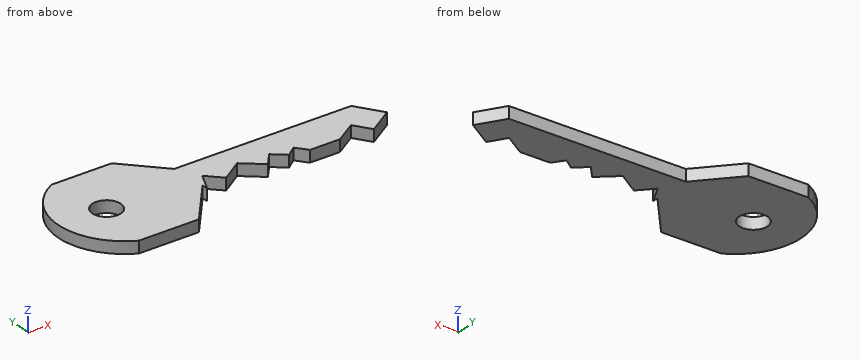
from build123d import *

# Parameters (mm, degrees)
F1_DEPTH = 2.5
F2_R     = 3
F3_DEPTH = 25


with BuildPart() as f1:
    # F0 (on Top) → F1 (new body)
    with BuildSketch(Plane.XY):
        with BuildLine():
            Line((18.500206, 13.484339), (5.681507, 13.484339))
            ThreePointArc((5.681507, 13.484339), (-2.025628, 0.984339), (5.681507, -11.515661))
            Line((5.681507, -11.515661), (18.500206, -11.515661))
            Line((18.500206, -11.515661), (26.226566, -2.179502))
            Line((26.226566, -2.179502), (26.226566, -3.515661))
            Line((26.226566, -3.515661), (28.245927, 0.636009))
            Line((28.245927, 0.636009), (31.124004, -2.351236))
            Line((31.124004, -2.351236), (35.732787, 0.682989))
            Line((35.732787, 0.682989), (39.747892, -2.72324))
            Line((39.747892, -2.72324), (42.058162, 0))
            Line((42.058162, 0), (44.656219, -2.204071))
            Line((44.656219, -2.204071), (46.799748, -0.583421))
            Line((46.799748, -0.583421), (48.568681, -2.923074))
            Line((48.568681, -2.923074), (54.981848, -2.923074))
            Line((54.981848, -2.923074), (59.484062, 0))
            Line((59.484062, 0), (61.766614, -3.515661))
            Line((61.766614, -3.515661), (67.18155, 0))
            Line((67.18155, 0), (63.620829, 5.484339))
            Line((63.620829, 5.484339), (25.8629, 5.484339))
            Line((25.8629, 5.484339), (18.500206, 13.484339))
        make_face()
    extrude(amount=F1_DEPTH)

    # F2 (on face) → F3 (cut)
    with BuildSketch(Plane.XY.offset(2.5)):
        with Locations((8.123178, 0.984339)):
            Circle(F2_R)
    extrude(amount=-F3_DEPTH, mode=Mode.SUBTRACT)


solid = f1.part
Design review of the part built by this model. Coordinates are the model's own, in mm. Give positions to 0.01 mm unless a question says otherwise; leave off trailing zeros. Write each loop counter-clockwise with the first axis right and the second up, starting at its lowest first coordinate (ties: lowest second). Pieces come first, ordered by that corner, then holes. Notation, with made-up numbers: M 77.25,0 L 131.25,0 A29 cw 131.25,27 Z; hole C -34,-36 d3. An arc over 180 degrees is marked long. Return JSON: item names as keys, results as strings. Group by question number.
Item 1: Clearance check with flat-ended pins moving along their axes: pin 1 Ø1 at (x, y) = (59.5, -3.5) entering from -Z; pin 2 Ø1.1 at (y, z) = (-2.5, 1.5) entering from -X; pin 3 Ø1.2 at (x, z) = (35.5, 1.5) entering from +Y. State where each tip first meets the part, or that it passes through.
Item 2: Wall thickness on line 1 along X through (y, z) = (0.5, 2.25); line 2 along Y through (x, z) = (53.5, 0.3); line 3 along X through (y, z) = (-2.5, 0.2): over which ranges is each line inside the solid? List them lowest first.
Item 3: Take a section at B-B (z = 1.5). Give the boundary of the cut face in (x, y).
Item 4: Take a section at C-C (x = 54). Give the boundary of the cut face in (y, z).
Item 5: Take a section at A-A (y = -1.25). Give the boundary of the cut face in (x, z), plus the area to 3 significant figures.
Item 6: Take a section at D-D (y = 11.25). Give the boundary of the cut face in (x, z), plus the area to 3 significant figures.
Return value:
{
 "1": {"pin 1": "passes through", "pin 2": "stops at x = -1.71", "pin 3": "stops at y = 5.48"},
 "2": {"line 1": "x = -2.02 to 5.16, 11.08 to 28.18, 28.38 to 35.45, 35.95 to 66.86", "line 2": "y = -2.92 to 5.48", "line 3": "x = -1.58 to 25.96, 26.23 to 26.72, 39.48 to 39.94, 48.25 to 55.63, 61.11 to 63.33"},
 "3": {"outline": "M 5.68,-11.52 L 18.5,-11.52 L 26.23,-2.18 L 26.23,-3.52 L 28.25,0.64 L 31.12,-2.35 L 35.73,0.68 L 39.75,-2.72 L 42.06,0 L 44.66,-2.2 L 46.8,-0.58 L 48.57,-2.92 L 54.98,-2.92 L 59.48,0 L 61.77,-3.52 L 67.18,0 L 63.62,5.48 L 25.86,5.48 L 18.5,13.48 L 5.68,13.48 A13.99 ccw Z; hole C 8.12,0.98 d6"},
 "4": {"outline": "M -2.92,0 L 5.48,0 L 5.48,2.5 L -2.92,2.5 Z"},
 "5": {"outline": "M -1.85,0 L 6.12,0 L 6.12,2.5 L -1.85,2.5 Z; M 10.13,0 L 27.33,0 L 27.33,2.5 L 10.13,2.5 Z; M 30.06,0 L 32.8,0 L 32.8,2.5 L 30.06,2.5 Z; M 38.01,0 L 41,0 L 41,2.5 L 38.01,2.5 Z; M 43.53,0 L 45.92,0 L 45.92,2.5 L 43.53,2.5 Z; M 47.3,0 L 57.56,0 L 57.56,2.5 L 47.3,2.5 Z; M 60.3,0 L 65.26,0 L 65.26,2.5 L 60.3,2.5 Z", "area": "121 mm2"},
 "6": {"outline": "M 2.46,0 L 20.56,0 L 20.56,2.5 L 2.46,2.5 Z", "area": "45.2 mm2"}
}
